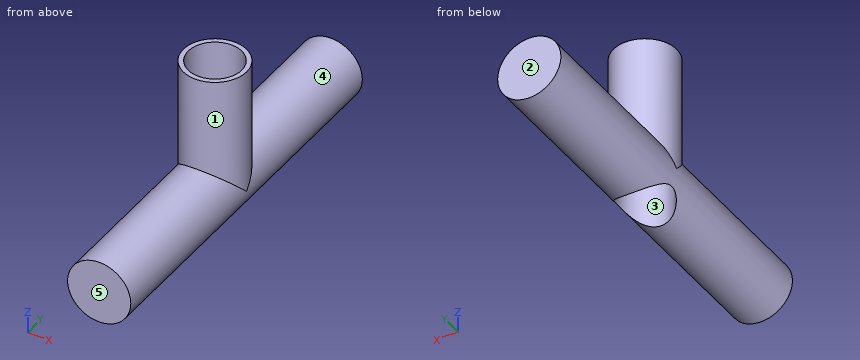
from build123d import *

# Parameters (mm, degrees)
F0_R     = 12.7
F1_DEPTH = 76.2
F2_R     = 12.7
F3_DEPTH = 50.8
F4_R     = 10.74617
F5_DEPTH = 63.501


with BuildPart() as f1:
    # F0 (on Front) → F1 (new body, symmetric)
    with BuildSketch(Plane.XZ):
        Circle(F0_R)
    extrude(amount=F1_DEPTH, both=True)

    # F2 (on Top) → F3 (join)
    with BuildSketch(Plane.XY):
        Circle(F2_R)
    extrude(amount=F3_DEPTH)

    # F4 (on face) → F5 (cut, through all)
    with BuildSketch(Plane.XY.offset(50.8)):
        Circle(F4_R)
    extrude(amount=-F5_DEPTH, mode=Mode.SUBTRACT)


solid = f1.part
Source: CAD feature listing. Evaluate the final solid. Frame: model axes, mm. Face numbers are marked on the shaded views. A direction names the side the tool comes from. Coordinates: 2 decimals unless noted, no trailing zeros. Order: outer loops, then holes, each group sorted by start corner. A loop starts at its lowest first (then second) coordinate and runs counter-clockwise, first axis right, second up. Notation, with made-up numbers: M -0.5,28.5 L 29.5,28.5 A27 cw 29.5,67.5 Z; hole C 11.25,77.25 d3. An arc over 180 degrees is marked long. Write each question's results on one line, items separated by ' | '. Start each with the question number.
Item 1: First-contact query: pin 1 Ø8 at (x, y) = (-6.5, 37.5) entering from +Z; pin 2 Ø3 at (x, z) = (8.5, 29.5) entering from -Y; pin 3 Ø1 at (x, y) = (3.5, 8.5) entering from -Z (3 decimals); pin 4 Ø12 at (x, y) = (7.5, -51.5) entering from +Z. Flat tips, straight axial feed; report the tip coordinate or a pass-through.
Item 2: Cut plane D-D (x = -8.5). Return loops of the section in (y, z), and give its area (3 significant figures).
Item 3: Cut plane C-C (z = 4). Return loops of the section in (x, y), and give its area (3 significant figures).
Item 4: Cut plane B-B (y = -6). Return loops of the section in (x, z), and give its area (3 significant figures).
Item 5: Draft query along Y for the marked faces 3, 4 and 5. Return one class per face: pulls with the +Y half, pulls with the -Y half, needs draft (parallel to the pull), parting line crosses it, or undercut.
Item 6: Cut plane A-A (x = 0). Return loops of the section in (y, z), and give its area (3 significant figures).
Item 7: Set-up query: the marked faces 1 and 2. Return all of +Z, -Z, +X, -X, +Y, -Y with unobstructed straight access to the full face (end or side cutting, diameter ignored); none if empty.
Item 8: Line query: probe 1 along Y at (x, z) = (0, 35); probe 2 along Y at (x, z) = (7.25, 27.5); probe 3 along X at (y, z) = (-21.5, 0.5). Output: solid intervals per line, ascending.
Checked values:
1) pin 1: stops at z = 12.45 | pin 2: stops at y = -10.6 | pin 3: passes through | pin 4: stops at z = 12.61
2) outline: M -76.2,-9.44 L -6.57,-9.44 L -6.57,50.8 L -9.44,50.8 L -9.44,9.44 L -76.2,9.44 Z; M 6.57,-9.44 L 76.2,-9.44 L 76.2,9.44 L 9.44,9.44 L 9.44,50.8 L 6.57,50.8 Z | area: 2,860 mm2
3) outline: M -12.05,-76.2 L 12.05,-76.2 L 12.05,-4 A12.7 ccw 12.05,4 L 12.05,76.2 L -12.05,76.2 L -12.05,4 A12.7 ccw -12.05,-4 Z; hole C 0,0 d21.49 | area: 3,320 mm2
4) outline: M -11.19,6 A12.7 ccw -8.92,-9.04 L -8.92,50.8 L -11.19,50.8 Z; M 8.92,-9.04 A12.7 ccw 11.19,6 L 11.19,50.8 L 8.92,50.8 Z | area: 291 mm2
5) face 3: undercut | face 4: needs draft | face 5: pulls with the -Y half
6) outline: M -76.2,-12.7 L -10.75,-12.7 L -10.75,50.8 L -12.7,50.8 L -12.7,12.7 L -76.2,12.7 Z; M 10.75,-12.7 L 76.2,-12.7 L 76.2,12.7 L 12.7,12.7 L 12.7,50.8 L 10.75,50.8 Z | area: 3,470 mm2
7) face 1: +Z | face 2: +Z, -Z, +X, -X, +Y
8) probe 1: y = -12.7 to -10.75, 10.75 to 12.7 | probe 2: y = -10.43 to -7.93, 7.93 to 10.43 | probe 3: x = -12.69 to 12.69
